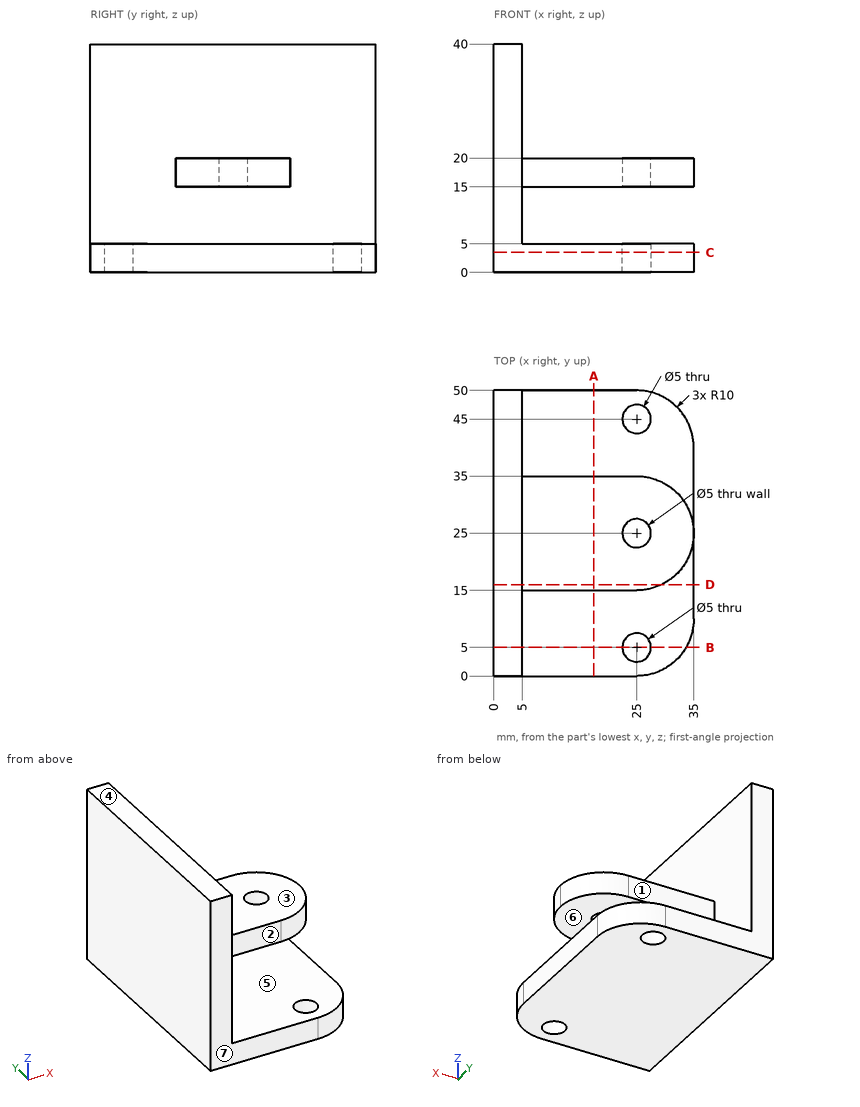
Answer from the drawing. Dimensions are ordinates in mm from the lowest x, y and z of the part. A direction names the side the tool comes from. Round coordinates to 2 decimals unless told otherwise and drop trailing zeros. Loops run counter-clockwise (first coordinate to the right, second up) from the corner with the lowest first, then second, coordinate; pieces in that order, holes last. Notation, with made-up numbers: M 11,40 L 19,40 A37 cw 19,79 Z; hole C -19,27 d2. An arc over 180 degrees is marked long. One line per question, with ' | ' between items. Start each with the question number.
(1) A cutting plane is placed at B-B on y = 5. Write down the section's boundary in (x, z).
(2) A cutting plane is placed at A-A on x = 17.5. Write down the section's boundary in (y, z), plus the area to 3 significant figures.
(3) A cutting plane is placed at D-D on y = 16. Write down the section's boundary in (x, z).
(4) For a pull along Z with two mould halves and no side action, classify the marked faces 4, 5, 6 and 7 as released by +Z, released by -Z, zero draft, split by the parting line, or undercut.
(5) A tool of negligible diameter and unlimited length cuts with its end or side. For the marked faces 1, 2 and 3, from which of +Z, -Z, +X, -X, +Y, -Y can it reach the whole face along a straight path? Write none if from no direction.
(6) Find the intervals of material crossed by line 1 (Y direction, x = 25, z = 3); line 2 (Z direction, x = 20, y = 24.5); line 3 (Y direction, x = 25, z = 17.4), in increasing order.
(7) A cutting plane is placed at C-C on z = 3.5. Write down the section's boundary in (x, y), plus the area to 3 significant figures.
(8) Flat-ended cylindrical pins translate along their axes: pin 1 Ø1.5 at (x, y) = (23, 43) entering from +Z; pin 2 Ø2 at (y, z) = (22, 15.5) entering from +X; pin 3 Ø1.5 at (x, z) = (12.5, 16.5) entering from -Y. Find the tip coordinate at first contact, or state that the pin passes through.
Geometry check:
1) outline: M 0,0 L 22.5,0 L 22.5,5 L 5,5 L 5,40 L 0,40 Z; M 27.5,0 L 33.66,0 L 33.66,5 L 27.5,5 Z
2) outline: M 0,0 L 50,0 L 50,5 L 0,5 Z; M 15,15 L 35,15 L 35,20 L 15,20 Z | area: 350 mm²
3) outline: M 0,0 L 35,0 L 35,5 L 5,5 L 5,15 L 29.36,15 L 29.36,20 L 5,20 L 5,40 L 0,40 Z
4) face 4: released by +Z | face 5: undercut | face 6: undercut | face 7: zero draft
5) face 1: +Z, +X, +Y | face 2: +Z, +X, -Y | face 3: +Z, +X, +Y, -Y
6) line 1: y = 0 to 2.5, 7.5 to 42.5, 47.5 to 50 | line 2: z = 0 to 5, 15 to 20 | line 3: y = 15 to 22.5, 27.5 to 35
7) outline: M 0,0 L 25,0 A10 ccw 35,10 L 35,40 A10 ccw 25,50 L 0,50 Z; hole C 25,5 d5; hole C 25,45 d5 | area: 1,670 mm²
8) pin 1: stops at z = 5 | pin 2: stops at x = 34.8 | pin 3: stops at y = 15
